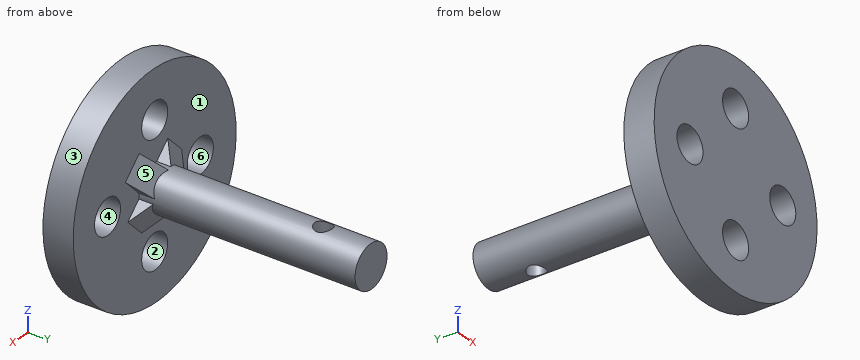
from build123d import *

# Parameters (mm, degrees)
SKETCH_1_R              = 12.5
EXTRUDE_1_DEPTH         = 3.5
SKETCH_2_R              = 2.45
EXTRUDE_2_DEPTH         = 25
SKETCH_4_R              = 2
CUT_EXTRUDE_1_DEPTH     = 31.618621785
SKETCH_4_5_R            = 2
CUT_EXTRUDE_2_DEPTH     = 31.618621785
RIB_1_REACH             = 35.537
SKETCH_8_WALL_W         = 74.969434882
SKETCH_8_WALL_H         = 3
RIB_6_REACH             = 35.537
SKETCH_9_WALL_W         = 75.07458535
SKETCH_9_WALL_H         = 3
RIB_7_REACH             = 35.537
SKETCH_11_WALL_W        = 75.144527038
SKETCH_11_WALL_H        = 3
CUT_EXTRUDE_4_OUTLINE_W = 1
CUT_EXTRUDE_4_OUTLINE_H = 4.900192031


# Read off the part's stored shape, not the designer's step: the extrude step
with BuildPart() as part:
    # Sketch 1 → Extrude 1 (new body)
    with BuildSketch(Plane(origin=(0, 0, 0), x_dir=(1, 0, 0), z_dir=(0, 1, 0))):
        with Locations(Location((0, 0, 0), (0, 0, 270))):
            Circle(SKETCH_1_R)
    extrude(amount=EXTRUDE_1_DEPTH)

    # Sketch 2 → Extrude 2 (add)
    with BuildSketch(Plane(origin=(0, 3.5, 0), x_dir=(1, 0, 0), z_dir=(0, 1, 0))):
        with Locations(Location((0, 0, 0), (0, 0, 270))):
            Circle(SKETCH_2_R)
    extrude(amount=EXTRUDE_2_DEPTH)

    # Sketch 4 → Cut-Extrude 1 (cut, through all)
    with BuildSketch(Plane(origin=(0, 3.5, 0), x_dir=(1, 0, 0), z_dir=(0, 1, 0))):
        with Locations(Location((0, 7, 0), (0, 0, 270))):
            Circle(SKETCH_4_R)
    extrude(amount=-CUT_EXTRUDE_1_DEPTH, mode=Mode.SUBTRACT)

    # Sketch 4_5 → Cut-Extrude 2 (cut, through all)
    with BuildSketch(Plane(origin=(0, 3.5, 0), x_dir=(1, 0, 0), z_dir=(0, 1, 0))):
        with Locations(Location((7.241500052, 0, 0), (0, 0, 270))):
            Circle(SKETCH_4_5_R)
        with Locations(Location((0, -7, 0), (0, 0, 270))):
            Circle(SKETCH_4_5_R)
        with Locations(Location((-7, 0, 0), (0, 0, 270))):
            Circle(SKETCH_4_5_R)
    extrude(amount=-CUT_EXTRUDE_2_DEPTH, mode=Mode.SUBTRACT)

    # Sketch 8 wall → Rib 1 (add, up to next)
    with BuildSketch(Plane(origin=(1.774725891, 4.95468166, 1.774725891), x_dir=(0.602127630795, -0.524294413919, 0.602127630795), z_dir=(0.37073213542, 0.85153706175, 0.37073213542)), mode=Mode.PRIVATE) as rib_1_sk1:
        Rectangle(SKETCH_8_WALL_W, SKETCH_8_WALL_H)
    rib_1_tool1 = extrude(rib_1_sk1.sketch, amount=-RIB_1_REACH, mode=Mode.PRIVATE) - part.part
    add(rib_1_tool1.solids().sort_by_distance((1.774725891, 4.95468166, 1.774725891))[0])

    # Sketch 9 wall → Rib 6 (add, up to next)
    with BuildSketch(Plane(origin=(-1.825339457, 4.971513253, -1.825339457), x_dir=(-0.608446485545, -0.509495582371, -0.608446485545), z_dir=(0.360267781279, -0.860473271836, 0.360267781279)), mode=Mode.PRIVATE) as rib_6_sk1:
        Rectangle(SKETCH_9_WALL_W, SKETCH_9_WALL_H)
    rib_6_tool1 = extrude(rib_6_sk1.sketch, amount=RIB_6_REACH, mode=Mode.PRIVATE) - part.part
    add(rib_6_tool1.solids().sort_by_distance((-1.825339457, 4.971513253, -1.825339457))[0])

    # Sketch 11 wall → Rib 7 (add, up to next)
    with BuildSketch(Plane(origin=(1.765395484, 4.77436806, -1.765395484), x_dir=(0.581684495472, -0.568582707664, -0.581684495472), z_dir=(0.402048688254, 0.822626102519, -0.402048688254)), mode=Mode.PRIVATE) as rib_7_sk1:
        Rectangle(SKETCH_11_WALL_W, SKETCH_11_WALL_H)
    rib_7_tool1 = extrude(rib_7_sk1.sketch, amount=-RIB_7_REACH, mode=Mode.PRIVATE) - part.part
    rib_7 = rib_7_tool1.solids().sort_by_distance((1.765395484, 4.77436806, -1.765395484))[0]
    add(rib_7)

    # Mirror 1: Rib 7 across plane
    add(rib_7.mirror(Plane(origin=(0, 0, 0), x_dir=(0.7071067811865465, 0, 0.7071067811865486), z_dir=(-0.7071067811865488, 0, 0.7071067811865464))))

    # Cut-Extrude 4 outline → Cut-Extrude 4 (revolve, cut)
    with BuildSketch(Plane.XZ.offset(-23)):
        with Locations((0.5, -9.238e-06)):
            Rectangle(CUT_EXTRUDE_4_OUTLINE_W, CUT_EXTRUDE_4_OUTLINE_H)
    revolve(axis=Axis((0, 23, 0), (0, 0, 1)), mode=Mode.SUBTRACT)


solid = part.part
Work out the finished part from the listing and answer in its coordinate system (mm). Face numbers are marked on the shaded views. A direction names the side the tool comes from. Round coordinates to 2 decimals unless told otherwise and drop trailing zeros. Write each loop counter-clockwise with the first axis right and the second up, starting at its lowest first coordinate (ties: lowest second). Pieces come first, ordered by that corner, then holes. Notation, with made-up numbers: M 85,11.25 L 90,11.25 A31 ccw 90,39.25 Z; hole C 44,43 d8. An arc over 180 degrees is marked long. Use a Markdown table: item, result.
1) The part is cut by section B-B on x = -7. Give the vertices of the cut face in (y, z), plus the area to 3 significant figures.
Taken from the geometry:
| item | result |
|---|---|
| outline | M 0,-10.36 L 3.5,-10.36 L 3.5,-2 L 0,-2 Z; M 0,2 L 3.5,2 L 3.5,10.36 L 0,10.36 Z |
| area | 58.5 mm2 |
2) Consider line 1 (Y direction, x = 0, z = -1.2); line 2 (X direction, y = 2.2, z = 0); line 3 (Z direction, x = -1, y = 3). Determine where each line is inside the solid, lowest interval first. Write a range as [from, to].
Taken from the geometry:
| item | result |
|---|---|
| line 1 | y = [0, 22], [24, 28.5] |
| line 2 | x = [-12.5, -9], [-5, 5.24], [9.24, 12.5] |
| line 3 | z = [-12.46, -8.73], [-5.27, 5.27], [8.73, 12.46] |
3) Determine the mould class of the marked faces 3, 4, 5 and 6 for opening direction X: pulls with the +X half, pulls with the -X half, needs draft (parallel to the pull), parting line crosses it, or undercut.
Taken from the geometry:
| item | result |
|---|---|
| face 3 | parting line crosses it |
| face 4 | undercut |
| face 5 | pulls with the +X half |
| face 6 | undercut |
4) The part is cut by section A-A on z = 7. Give the vertices of the cut face in (x, y), plus the area to 3 significant figures.
Taken from the geometry:
| item | result |
|---|---|
| outline | M -10.36,0 L -2,0 L -2,3.5 L -10.36,3.5 Z; M 2,0 L 10.36,0 L 10.36,3.5 L 2,3.5 Z |
| area | 58.5 mm2 |
5) Flat-ended cylindrical pins translate along their axes: pin 1 (2 mm diameter, centred on x = 6, z = 10, fed in from +Y); pin 2 (10 mm diameter, centred on y = 6, z = 3, fed in from +X); pin 3 (5 mm diameter, centred on y = 23.5, z = 4.5, fed in from +X). Find the tip coordinate at first contact, or state that the pin passes through.
Taken from the geometry:
| item | result |
|---|---|
| pin 1 | stops at y = 3.5 |
| pin 2 | stops at x = 12.5 |
| pin 3 | stops at x = 1.42 |
6) The part is cut by section C-C on x = 1.5. Give the vertices of the cut face in (y, z), plus the area to 3 significant figures.
Taken from the geometry:
| item | result |
|---|---|
| outline | M 0,-12.41 L 3.5,-12.41 L 3.5,-8.32 L 0,-8.32 Z; M 0,-5.68 L 3.5,-5.68 L 3.5,-3.62 L 4,-3.62 L 4.82,-1.94 L 28.5,-1.94 L 28.5,1.94 L 5,1.94 L 4.27,3.62 L 3.5,3.62 L 3.5,5.68 L 0,5.68 Z; M 0,8.32 L 3.5,8.32 L 3.5,12.41 L 0,12.41 Z |
| area | 169 mm2 |
7) The part is cut by section D-D on z = 10. Give the vertices of the cut face in (x, y), plus the area to 3 significant figures.
Taken from the geometry:
| item | result |
|---|---|
| outline | M -7.5,0 L 7.5,0 L 7.5,3.5 L -7.5,3.5 Z |
| area | 52.5 mm2 |
8) Which of the six approach directions +Z, -Z, +X, -X, +Y, -Y give full straight-line access (tool end or side, diameter ignored) to the marked faces 1 and 2?
Taken from the geometry:
| item | result |
|---|---|
| face 1 | +Y |
| face 2 | +Y, -Y |
